For this review, take the finished solid that the model builds, in its own axes (mm). Round coordinates to 2 decimals unless told otherwise and drop trailing zeros. Write each loop counter-clockwise with the first axis right and the second up, starting at its lowest first coordinate (ties: lowest second). Pieces come first, ordered by that corner, then holes. Notation, with made-up numbers: (17.5, -13.5) -> (69.5, -13.5) arc R26 ccw to (69.5, 24.5) -> close; hole circle Ø2 at (-2, 58). An arc over 180 degrees is marked (long way). Write each question's results on one line, items separated by ' | '. Start each with the question number.
Item 1: Add section B-B (z = 2.35). Count the separate pieces of the cut face and the enclosed holes in it, plus the area to 3 significant figures.
Item 2: Clearance check with a flat-ended pin moving along its axis: pin 1 (4 mm diameter, centred on x = 100, y = 15, fed in from -Z). State where the tip first meets the part, or that it passes through.
Item 3: Add section A-A (x = -30). State the section outline as (y, z) points, plus the area to 3 significant figures.
Item 4: To check wall thickness, follow line 1 along Y through (x, z) = (-100, 4.05); line 2 along Y through (x, z) = (-54, 4.5); line 3 along Y through (x, z) = (-50, 3.75). State the ranges of each line that lie inside material, in increasing order.
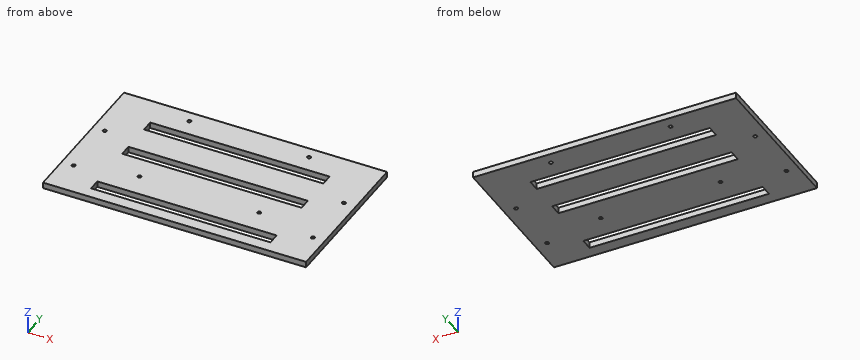
from build123d import *

# Parameters (mm, degrees)
SKETCH_1_W          = 220
SKETCH_1_H          = 130
EXTRUDE_1_DEPTH     = 5
SKETCH_2_R          = 1.5
CUT_EXTRUDE_1_DEPTH = 5
SKETCH_3_R          = 1.5
CUT_EXTRUDE_2_DEPTH = 5
SKETCH_4_W          = 150
SKETCH_4_H          = 10
CUT_EXTRUDE_3_DEPTH = 10


with BuildPart() as part:
    # 草图1 → 凸台-拉伸1 (new body)
    with BuildSketch(Plane.XY):
        Rectangle(SKETCH_1_W, SKETCH_1_H)
    extrude(amount=EXTRUDE_1_DEPTH)

    # 草图2 → 切除-拉伸1 (cut)
    with BuildSketch(Plane.XY.offset(5)):
        with Locations((-50, 55)):
            Circle(SKETCH_2_R)
        with Locations((50, 55)):
            Circle(SKETCH_2_R)
        with Locations((50, -25)):
            Circle(SKETCH_2_R)
        with Locations((-50, -25)):
            Circle(SKETCH_2_R)
    extrude(amount=-CUT_EXTRUDE_1_DEPTH, mode=Mode.SUBTRACT)

    # 草图3 → 切除-拉伸2 (cut)
    with BuildSketch(Plane.XY.offset(5)):
        with Locations((100, 15)):
            Circle(SKETCH_3_R)
        with Locations((100, -35)):
            Circle(SKETCH_3_R)
        with Locations((-100, 15)):
            Circle(SKETCH_3_R)
        with Locations((-100, -35)):
            Circle(SKETCH_3_R)
    extrude(amount=-CUT_EXTRUDE_2_DEPTH, mode=Mode.SUBTRACT)

    # 草图4 → 切除-拉伸3 (cut)
    with BuildSketch(Plane.XY.offset(5)):
        Rectangle(SKETCH_4_W, SKETCH_4_H)
        with Locations((0, 35)):
            Rectangle(SKETCH_4_W, SKETCH_4_H)
        with Locations((0, -50)):
            Rectangle(SKETCH_4_W, SKETCH_4_H)
    extrude(amount=-CUT_EXTRUDE_3_DEPTH, mode=Mode.SUBTRACT)


solid = part.part
Responses:
1) separate pieces: 1 | enclosed holes: 11 | area: 24,000 mm^2
2) pin 1: stops at z = 0
3) outline: (-65, 0) -> (-55, 0) -> (-55, 5) -> (-65, 5) -> close; (-45, 0) -> (-5, 0) -> (-5, 5) -> (-45, 5) -> close; (5, 0) -> (30, 0) -> (30, 5) -> (5, 5) -> close; (40, 0) -> (65, 0) -> (65, 5) -> (40, 5) -> close | area: 500 mm^2
4) line 1: y = -65 to -36.5, -33.5 to 13.5, 16.5 to 65 | line 2: y = -65 to -55, -45 to -5, 5 to 30, 40 to 65 | line 3: y = -65 to -55, -45 to -26.5, -23.5 to -5, 5 to 30, 40 to 53.5, 56.5 to 65
